from build123d import *

# Parameters (mm, degrees)
F3_SIZE = 5.08


# Not quite as in the source:
# - a fillet or chamfer that OpenCascade refuses, or shapes differently, is made with other operations: its cross-section is extruded or revolved along the edge and cut away or added


with BuildPart() as f1:
    # F0 (on Front) → F1 (revolve)
    with BuildSketch(Plane.XZ):
        Polygon((32.8848399222, 52.7038350701), (13.7998890132, 52.7038350701), (13.7998890132, 35.9677970409), (6.1659086496, 35.9677970409), (6.1659086496, 46.2443120778), (0, 46.2443120778), (0, 0), (32.8848399222, 7.1935597807), align=None)
    revolve(axis=Axis((0, 0, 23.1221560389), (0, 0, -1)))

    # F2: chamfer of 5.08 on 3 edges, made by hand

    # F2_s1 → F2_t2 (revolve, cut)
    with BuildSketch(Plane.XZ):
        Polygon((28.8904202174, 6.319780343), (32.8848399222, 11.2824323984), (32.8848399222, 7.1935597807), align=None)
    revolve(axis=Axis((0, 0, 7.1935597807), (0, 0, -1)), mode=Mode.SUBTRACT)

    # F2_s3 → F2_t4 (revolve, cut)
    with BuildSketch(Plane.XZ):
        Polygon((27.8048399222, 52.7038350701), (32.8848399222, 47.6238350701), (32.8848399222, 52.7038350701), align=None)
    revolve(axis=Axis((0, 0, 52.7038350701), (0, 0, -1)), mode=Mode.SUBTRACT)

    # F3
    f3_edges = [f1.edges().sort_by_distance(p)[0] for p in [
        (14.44521, 0, 3.15989),
        (-28.89042, 0, 6.31978),
    ]]
    chamfer(f3_edges, length=F3_SIZE)


solid = f1.part
Input: part model. Units: mm. Frame: model coordinates. A direction names the side the tool comes from. Round coordinates to 2 decimals unless told otherwise and drop trailing zeros. Order: outer loops, then holes, each group sorted by start corner. A loop starts at its lowest first (then second) coordinate and runs counter-clockwise, first axis right, second up. Notation, with made-up numbers: (54, 28.25) - (103, 28.25) arc R19 ccw to (103, 44.25) - close; hole circle Ø3 at (-15, 48). An arc over 180 degrees is marked (long way). Use a Markdown table: item, result.
1. Mould query, pull axis Y, two halves, no side actions, for faces 1 (the face through (6, -13, 52.704)), 2 (the face through (-26.096, 20.01, 29.708)), 3 (the face through (-2.992, 13.472, 44.219)). Classes: +Y half, -Y half, draft (parallel to the pull), parting line (faces both ways), or undercut.
Evaluation:
| item | result |
|---|---|
| face 1 | draft |
| face 2 | parting line |
| face 3 | undercut |
2. First-contact query: pin 1 (12 mm diameter, centred on x = 17, z = 21, fed in from -Y); pin 2 (1.5 mm diameter, centred on y = 18, z = 41, fed in from -X); pin 3 (8 mm diameter, centred on x = -25.5, z = 47.5, fed in from -Y). Flat tips, straight axial feed; report the tip coordinate or a pass-through.
Evaluation:
| item | result |
|---|---|
| pin 1 | y = -30.99 |
| pin 2 | x = -28 |
| pin 3 | y = -24.88 |
3. Material intervals for probe 1 along Y at (x, z) = (0, 41); probe 2 along Y at (x, z) = (-5, 36), sorted ascending.
Evaluation:
| item | result |
|---|---|
| probe 1 | -32.88 to -13.8, -6.17 to 6.17, 13.8 to 32.88 |
| probe 2 | -32.5 to -12.86, -3.61 to 3.61, 12.86 to 32.5 |
4. Access query for faces 4 (the face through (-0.324, 1.461, 0.327)), 5 (the face through (-1.34, 6.02, 41.18)). Directions: +Z, -Z, +X, -X, +Y, -Y. A direction counts if a zero-diameter tool reaches every point of the face in a straight line with its end or side. Return the directions, or none.
Evaluation:
| item | result |
|---|---|
| face 4 | -Z |
| face 5 | +Z |
5. Section A-A on z = 35. Return the cut outline in (x, y), then the cut area to 3 significant figures.
Evaluation:
| item | result |
|---|---|
| outline | circle Ø65.77 at (0, 0) |
| area | 3,400 mm^2 |
